For this review, take the finished solid that the model builds, in its own axes (mm). Face numbers are marked on the shaded views. Round coordinates to 2 decimals unless told otherwise and drop trailing zeros. Order: outer loops, then holes, each group sorted by start corner. A loop starts at its lowest first (then second) coordinate and runs counter-clockwise, first axis right, second up. Notation, with made-up numbers: (-10, 4) - (-5, 4) arc R30 cw to (-5, 31) - close; hole circle Ø5 at (-31.5, -15.75). An arc over 180 degrees is marked (long way). Write each question's results on one line, items separated by ' | '. Start each with the question number.
(1) Take a section at B-B, the plane y = -15.24. Give the boundary of the cut face in (x, z) (3 decimals).
(2) Take a section at C-C, the plane x = 15.24. Give the boundary of the cut face in (y, z) (3 decimals).
(3) For L1, parallel to Y at x = 6, z = 1.9; L2, parallel to Y at x = 8, z = 1.3; L3, parallel to X at y = -5.5, z = 0.55, list the stretches that pass through material, from the lowest coordinate up. Write a range as from..to.
(4) Take a section at A-A, the plane z = 0.8. Give the boundary of the cut face in (x, y) (3 decimals).
(5) Insertion check: pin 1 Ø1.5 at (x, y) = (5.5, -4.5) entering from -Z. The pin has a flat end and moves straight along its axis. Give the tip position at first contact, or say it passes through.
(6) Draft analysis for pull direction X (two halves, no side actions). For the marked faces 1 and 2, state which applies: pulls with the +X half, pulls with the -X half, needs draft (parallel to the pull), parting line crosses it, or undercut.
(7) Take a section at D-D, the plane y = -23.5. Give the boundary of the cut face in (x, z), plus the area to 3 significant figures.
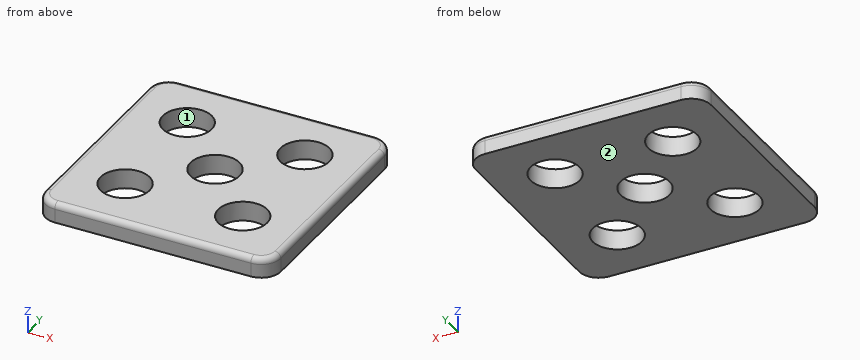
```python
from build123d import *

# Parameters (mm, degrees)
F0_R     = 3.175
F1_DEPTH = 2.54
F2_R     = 0.762


with BuildPart() as f1:
    # F0 (on Top) → F1 (new body)
    with BuildSketch(Plane.XY):
        with BuildLine():
            Line((27.94, 0), (2.54, 0))
            ThreePointArc((2.54, 0), (0.743949, -0.743949), (0, -2.54))
            Line((0, -2.54), (0, -27.94))
            ThreePointArc((0, -27.94), (0.743949, -29.736051), (2.54, -30.48))
            Line((2.54, -30.48), (27.94, -30.48))
            ThreePointArc((27.94, -30.48), (29.736051, -29.736051), (30.48, -27.94))
            Line((30.48, -27.94), (30.48, -2.54))
            ThreePointArc((30.48, -2.54), (29.736051, -0.743949), (27.94, 0))
        make_face()
        with Locations((7.62, -22.86)):
            Circle(F0_R, mode=Mode.SUBTRACT)
        with Locations((22.86, -22.86)):
            Circle(F0_R, mode=Mode.SUBTRACT)
        with Locations((15.24, -15.24)):
            Circle(F0_R, mode=Mode.SUBTRACT)
        with Locations((7.62, -7.62)):
            Circle(F0_R, mode=Mode.SUBTRACT)
        with Locations((22.86, -7.62)):
            Circle(F0_R, mode=Mode.SUBTRACT)
    extrude(amount=F1_DEPTH)

    # F2
    f2_edges = [f1.edges().sort_by_distance(p)[0] for p in [
        (30.48, -15.24, 2.54),
    ]]
    fillet(f2_edges, radius=F2_R)


solid = f1.part
```
Results below:
1) outline: (0, 0) - (12.065, 0) - (12.065, 2.54) - (0.762, 2.54) arc R0.762 ccw to (0, 1.778) - close; (18.415, 0) - (30.48, 0) - (30.48, 1.778) arc R0.762 ccw to (29.718, 2.54) - (18.415, 2.54) - close
2) outline: (-30.48, 0) - (-18.415, 0) - (-18.415, 2.54) - (-29.718, 2.54) arc R0.762 ccw to (-30.48, 1.778) - close; (-12.065, 0) - (0, 0) - (0, 1.778) arc R0.762 ccw to (-0.762, 2.54) - (-12.065, 2.54) - close
3) L1: y = -30.47..-25.59, -20.13..-10.35, -4.89..-0.01 | L2: y = -30.48..-26.01, -19.71..-10.77, -4.47..0 | L3: x = 0..5.26, 9.98..20.5, 25.22..30.48
4) outline: (0, -27.94) arc R2.54 ccw to (2.54, -30.48) - (27.94, -30.48) arc R2.54 ccw to (30.48, -27.94) - (30.48, -2.54) arc R2.54 ccw to (27.94, 0) - (2.54, 0) arc R2.54 ccw to (0, -2.54) - close; hole circle Ø6.35 at (7.62, -22.86); hole circle Ø6.35 at (7.62, -7.62); hole circle Ø6.35 at (15.24, -15.24); hole circle Ø6.35 at (22.86, -22.86); hole circle Ø6.35 at (22.86, -7.62)
5) pin 1: stops at z = 0
6) face 1: undercut | face 2: needs draft
7) outline: (0, 0) - (4.51, 0) - (4.51, 2.54) - (0.76, 2.54) arc R0.76 ccw to (0, 1.78) - close; (10.73, 0) - (19.75, 0) - (19.75, 2.54) - (10.73, 2.54) - close; (25.97, 0) - (30.48, 0) - (30.48, 1.78) arc R0.76 ccw to (29.72, 2.54) - (25.97, 2.54) - close | area: 45.6 mm^2
